```python
from build123d import *

# Parameters (mm, degrees)
F1_DEPTH = 51
F3_DEPTH = 10
F5_DEPTH = 10


with BuildPart() as f1:
    # F0 (on Right) → F1 (new body, symmetric)
    with BuildSketch(Plane.YZ):
        Polygon((-51, -11.5), (51, -11.5), (51, 11.5), (-42, 11.5), align=None)
    extrude(amount=F1_DEPTH, both=True)

    # F2 (on face) → F3 (cut)
    with BuildSketch(Plane(origin=(0, 51, 0), x_dir=(-1, 0, 0), z_dir=(0, 1, 0))):
        Polygon((-3.535534, -3.535534), (0, -5), (3.535534, -3.535534), (5, 0), (3.535534, 3.535534), (0, 5), (-3.535534, 3.535534), (-5, 0), align=None)
        Polygon((33.535534, 3.535534), (30, 5), (26.464466, 3.535534), (25, 0), (26.464466, -3.535534), (30, -5), (33.535534, -3.535534), (35, 0), align=None)
        Polygon((-25, 0), (-26.464466, 3.535534), (-30, 5), (-33.535534, 3.535534), (-35, 0), (-33.535534, -3.535534), (-30, -5), (-26.464466, -3.535534), align=None)
    extrude(amount=-F3_DEPTH, mode=Mode.SUBTRACT)

    # F4 (on face) → F5 (cut)
    with BuildSketch(Plane(origin=(-51, 0, 0), x_dir=(0, -1, 0), z_dir=(-1, 0, 0))):
        Polygon((-3.535534, -3.535534), (0, -5), (3.535534, -3.535534), (5, 0), (3.535534, 3.535534), (0, 5), (-3.535534, 3.535534), (-5, 0), align=None)
        Polygon((33.535534, 3.535534), (30, 5), (26.464466, 3.535534), (25, 0), (26.464466, -3.535534), (30, -5), (33.535534, -3.535534), (35, 0), align=None)
        Polygon((-25, 0), (-26.464466, 3.535534), (-30, 5), (-33.535534, 3.535534), (-35, 0), (-33.535534, -3.535534), (-30, -5), (-26.464466, -3.535534), align=None)
    extrude(amount=-F5_DEPTH, mode=Mode.SUBTRACT)


solid = f1.part
```
CAD build for the part. Positions are in the model's coordinates, mm. A direction names the side the tool comes from. Round coordinates to 2 decimals unless told otherwise and drop trailing zeros. Order: outer loops, then holes, each group sorted by start corner. A loop starts at its lowest first (then second) coordinate and runs counter-clockwise, first axis right, second up.
Item 1: Probe line 1 along X through (y, z) = (30, 4.75); line 2 along Y through (x, z) = (43.5, 8.5); line 3 along Y through (x, z) = (24, -4.5). List the from-to ranges inside material, lowest first.
Item 2: Pin check, flat tips, straight feed: pin 1 (6 mm diameter, centred on x = -21.5, z = -1, fed in from -Y); pin 2 (3 mm diameter, centred on y = 31, z = -1.5, fed in from -X); pin 3 (5 mm diameter, centred on x = -28.5, z = -0.5, fed in from +Y). Stop position of each tip, or through.
Item 3: Tool access for faces 1 (the face through (-28.26, 46.07, 4.28)), 2 (the face through (1, 51, -5)), 3 (the face through (-46.07, -34.26, -1.79)): list every direction of +Z, -Z, +X, -X, +Y, -Y with a clear straight run to the whole face (end or side of a thin tool).
Item 4: Saw through at C-C on z = -7.25. Write the cut outline in (x, y).
Item 5: Saw through at B-B on x = -6.5. Write the cut outline in (y, z), then the cut area to 3 significant figures.
Item 6: Saw through at A-A on z = -1.75. Write the cut outline in (x, y), then the cut area to 3 significant figures.
Item 7: Mould opens along Y. For faces 4 (the face through (-46.07, -28.21, -4.26)), 5 (the face through (30, 41, 0)), 6 (the face through (-46.07, -1.74, -4.28)), 7 (the face through (-1.74, 46.07, -4.28)) say: pulls with the +Y half, pulls with the -Y half, needs draft (parallel to the pull), parting line crosses it, or undercut.
Reported:
1. line 1: x = -41 to 51
1. line 2: y = -43.17 to 51
1. line 3: y = -48.26 to 51
2. pin 1: stops at y = -48.07
2. pin 2: stops at x = -41
2. pin 3: stops at y = 41
3. face 1: +Y
3. face 2: +Z, -Z, +X, -X, +Y
3. face 3: -X
4. outline: (-51, -49.34) - (51, -49.34) - (51, 51) - (-51, 51) - close
5. outline: (-51, -11.5) - (51, -11.5) - (51, 11.5) - (-42, 11.5) - close
5. area: 2,240 mm2
6. outline: (-51, -47.18) - (51, -47.18) - (51, 51) - (34.28, 51) - (34.28, 41) - (25.72, 41) - (25.72, 51) - (4.28, 51) - (4.28, 41) - (-4.28, 41) - (-4.28, 51) - (-25.72, 51) - (-25.72, 41) - (-34.28, 41) - (-34.28, 51) - (-51, 51) - (-51, 34.28) - (-41, 34.28) - (-41, 25.72) - (-51, 25.72) - (-51, 4.28) - (-41, 4.28) - (-41, -4.28) - (-51, -4.28) - (-51, -25.72) - (-41, -25.72) - (-41, -34.28) - (-51, -34.28) - close
6. area: 9,500 mm2
7. face 4: undercut
7. face 5: pulls with the +Y half
7. face 6: undercut
7. face 7: needs draft
